Geometry check sheet. Reference: the model listing, model coordinates, mm. A direction names the side the tool comes from. Coordinates: 2 decimals unless noted, no trailing zeros. Write each loop counter-clockwise with the first axis right and the second up, starting at its lowest first coordinate (ties: lowest second). Pieces come first, ordered by that corner, then holes. Notation, with made-up numbers: (40, 74) -> (51, 74) arc R18 ccw to (51, 102) -> close; hole circle Ø8 at (88.25, -18.75). An arc over 180 degrees is marked (long way). One line per question, with ' | ' between items.
from build123d import *

# Parameters (mm, degrees)
PAD004_DEPTH         = 3
SKETCH049_R          = 1.2
POCKET025_DEPTH      = 3.001
PAD003_DEPTH         = 1
SKETCH048_R          = 1.2
POCKET023_DEPTH      = 4.001
POCKET023_DEPTH_BACK = 0.001
POCKET024_DEPTH      = 1.75
SKETCH052_R          = 2.1
POCKET026_DEPTH      = 2.4


with BuildPart() as part:
    # Sketch047 → Pad004 (new body)
    with BuildSketch(Plane.XY):
        with BuildLine():
            Line((-6.5, 0), (6.5, 0))
            ThreePointArc((6.5, 0), (7.914214, 0.585786), (8.5, 2))
            Line((8.5, 2), (8.5, 25))
            ThreePointArc((8.5, 25), (7.914214, 26.414214), (6.5, 27))
            Line((6.5, 27), (-6.5, 27))
            ThreePointArc((-6.5, 27), (-7.914214, 26.414214), (-8.5, 25))
            Line((-8.5, 25), (-8.5, 2))
            ThreePointArc((-8.5, 2), (-7.914214, 0.585786), (-6.5, 0))
        make_face()
    extrude(amount=-PAD004_DEPTH)

    # Sketch049 → Pocket025 (cut, through all)
    with BuildSketch(Plane.XY):
        with Locations((-5.5, 24)):
            Circle(SKETCH049_R)
        with Locations((5.5, 24)):
            Circle(SKETCH049_R)
        with Locations((5.5, 3)):
            Circle(SKETCH049_R)
        with Locations((-5.5, 3)):
            Circle(SKETCH049_R)
    extrude(amount=-POCKET025_DEPTH, mode=Mode.SUBTRACT)

    # Sketch051 (on DatumPlane) → Pad003 (join)
    with BuildSketch(Plane.XY.offset(-3)):
        with BuildLine():
            ThreePointArc((-3.962007, 20.45), (-8, 13.5), (-3.962007, 6.55))
            ThreePointArc((-2.971505, 5.0875), (-3.296554, 5.934022), (-3.962007, 6.55))
            ThreePointArc((-2.971505, 5.0875), (0, 2.5), (2.971505, 5.0875))
            ThreePointArc((3.962007, 6.55), (3.296554, 5.934022), (2.971505, 5.0875))
            ThreePointArc((3.962007, 6.55), (8, 13.5), (3.962007, 20.45))
            ThreePointArc((2.971505, 21.9125), (3.296554, 21.065978), (3.962007, 20.45))
            ThreePointArc((2.971505, 21.9125), (0, 24.5), (-2.971505, 21.9125))
            ThreePointArc((-3.962007, 20.45), (-3.296554, 21.065978), (-2.971505, 21.9125))
        make_face()
    extrude(amount=-PAD003_DEPTH)

    # Sketch048 → Pocket023 (cut, two sides)
    with BuildSketch(Plane.XY) as pocket023_sk:
        with Locations((0, 5.5)):
            Circle(SKETCH048_R)
        with Locations((0, 21.5)):
            Circle(SKETCH048_R)
    extrude(amount=-POCKET023_DEPTH, mode=Mode.SUBTRACT)
    extrude(pocket023_sk.sketch, amount=POCKET023_DEPTH_BACK, mode=Mode.SUBTRACT)

    # Sketch050 → Pocket024 (cut)
    with BuildSketch(Plane.XY):
        Polygon((4.287564, 0.9), (6.712436, 0.9), (7.924871, 3), (6.712436, 5.1), (4.287564, 5.1), (3.075129, 3), align=None)
        Polygon((6.712436, 26.1), (4.287564, 26.1), (3.075129, 24), (4.287564, 21.9), (6.712436, 21.9), (7.924871, 24), align=None)
        Polygon((-4.287564, 21.9), (-3.075129, 24), (-4.287564, 26.1), (-6.712436, 26.1), (-7.924871, 24), (-6.712436, 21.9), align=None)
        Polygon((-4.287564, 0.9), (-3.075129, 3), (-4.287564, 5.1), (-6.712436, 5.1), (-7.924871, 3), (-6.712436, 0.9), align=None)
    extrude(amount=-POCKET024_DEPTH, mode=Mode.SUBTRACT)

    # Sketch052 → Pocket026 (cut)
    with BuildSketch(Plane.XY):
        with Locations((0, 21.5)):
            Circle(SKETCH052_R)
        with Locations((0, 5.5)):
            Circle(SKETCH052_R)
    extrude(amount=-POCKET026_DEPTH, mode=Mode.SUBTRACT)


solid = part.part
1. Cross-section at C-C on z = -3.3. Record the boundary of the cut face in (x, y), and give its area (3 significant figures).
Worked answers:
outline: (-3.96, 6.55) arc R2 cw to (-2.97, 5.09) arc R3 ccw to (2.97, 5.09) arc R2 cw to (3.96, 6.55) arc R8 ccw to (3.96, 20.45) arc R2 cw to (2.97, 21.91) arc R3 ccw to (-2.97, 21.91) arc R2 cw to (-3.96, 20.45) arc R8 ccw to start; hole circle Ø2.4 at (0, 5.5); hole circle Ø2.4 at (0, 21.5) | area: 223 mm²
2. Material ranges on line 1 (Y direction, x = 0, z = -1.3); line 2 (Y direction, x = 5.5, z = -2.65); line 3 (X direction, y = 3.75, z = -1.65), recorded low to high. Write a range as from..to.
Worked answers:
line 1: 0..3.4, 7.6..19.4, 23.6..27 | line 2: 0..1.8, 4.2..22.8, 25.2..27 | line 3: -8.5..-7.49, -3.51..-1.16, 1.16..3.51, 7.49..8.5
3. Cross-section at A-A on x = 0. Record the boundary of the cut face in (y, z).
Worked answers:
outline: (0, -3) -> (2.5, -3) -> (2.5, -4) -> (4.3, -4) -> (4.3, -2.4) -> (3.4, -2.4) -> (3.4, 0) -> (0, 0) -> close; (6.7, -4) -> (20.3, -4) -> (20.3, -2.4) -> (19.4, -2.4) -> (19.4, 0) -> (7.6, 0) -> (7.6, -2.4) -> (6.7, -2.4) -> close; (22.7, -4) -> (24.5, -4) -> (24.5, -3) -> (27, -3) -> (27, 0) -> (23.6, 0) -> (23.6, -2.4) -> (22.7, -2.4) -> close
4. Cross-section at D-D on y = 21.5. Record the boundary of the cut face in (x, z), and give its area (3 significant figures).
Worked answers:
outline: (-8.5, -3) -> (-3.07, -3) -> (-3.07, -4) -> (-1.2, -4) -> (-1.2, -2.4) -> (-2.1, -2.4) -> (-2.1, 0) -> (-8.5, 0) -> close; (1.2, -4) -> (3.07, -4) -> (3.07, -3) -> (8.5, -3) -> (8.5, 0) -> (2.1, 0) -> (2.1, -2.4) -> (1.2, -2.4) -> close | area: 43.2 mm²
5. Tool access check on faces 5 (the face through (7, 4, -1.75)), 6 (the face through (8.5, 13, -1)), 7 (the face through (-8, 13.6, -3.5)). Record the directions out of +Z, -Z, +X, -X, +Y, -Y that give a thin tool (end or side, any length) a straight path to the whole face; none if there is none.
Worked answers:
face 5: +Z | face 6: +Z, -Z, +X, +Y, -Y | face 7: -Z, -X
6. Cross-section at B-B on z = -0.8. Give the number of separate pieces and of enclosed holes in the cut face, and give its area (3 significant figures).
Worked answers:
separate pieces: 1 | enclosed holes: 6 | area: 367 mm²
7. Mould release check, pull along X, two halves, no side actions. Record for faces 1 (the face through (-7.31, 25.065, -0.863)), 2 (the face through (0, 27, -1)), 3 (the face through (3.673, 1.965, -0.863)), 4 (the face through (8, 13.4, -3.5)): released by +X, released by -X, zero draft, split by the parting line, or undercut.
Worked answers:
face 1: undercut | face 2: zero draft | face 3: undercut | face 4: released by +X
8. Go/stop test with flat-tipped pins: P1, Ø1.3, axis at x = -6, y = 23, coming from the +Z side; P2, Ø1.4, axis at x = 0, y = 21.5, coming from the +Z side; P3, Ø1.5, axis at x = -4, y = 21.5, coming from the -Z side; P4, Ø2, axis at x = 0.5, y = 5, coming from the +Z side. Record where each tip stops, or that it passes through.
Worked answers:
P1: z = -1.75 | P2: through | P3: z = -3 | P4: z = -2.4
